Read the model definition and answer for the solid it produces. Units are mm, in the model's axes. A direction names the side the tool comes from. Round coordinates to 2 decimals unless told otherwise and drop trailing zeros. Loops run counter-clockwise (first coordinate to the right, second up) from the corner with the lowest first, then second, coordinate; pieces in that order, holes last. Notation, with made-up numbers: M 69.25,14.5 L 124.25,14.5 A29 cw 124.25,44.5 Z; hole C 58.5,-36 d5. An arc over 180 degrees is marked long. Write each question's results on one line, items separated by ' | '.
from build123d import *

# Parameters (mm, degrees)
SKETCH_1_W                     = 55
SKETCH_1_H                     = 60
EXTRUDE_1_DEPTH                = 16.5
HOLE_WIZARD_3_6_3_6_1_D        = 3.6
HOLE_WIZARD_3_6_3_6_1_DEPTH    = 25
HOLE_WIZARD_3_6_3_6_1_TIP      = 1.081549114
HOLE_WIZARD_M2_5_1_D           = 2.05
HOLE_WIZARD_M2_5_1_DEPTH       = 14
HOLE_WIZARD_M2_5_1_TIP         = 0.615882135
SKETCH_8_W                     = 35
SKETCH_8_H                     = 20.4
CUT_EXTRUDE_1_DEPTH            = 44.914690025
CUT_EXTRUDE_START              = 2.5
SKETCH_9_W                     = 20
SKETCH_9_H                     = 6
CUT_EXTRUDE_2_DEPTH            = 42.414690025
SHELL_START                    = 1.8
SHELL_1_DEPTH                  = 14.7
EXTRUDE_2_DEPTH                = 3
HOLE_WIZARD_1_AT_2_COUNT       = 2
HOLE_WIZARD_1_AT_2_PITCH       = 48
HOLE_WIZARD_1_AT_3_COUNT       = 2
HOLE_WIZARD_1_AT_3_PITCH       = 27.5
HOLE_WIZARD_1_AT_4_COUNT       = 2
HOLE_WIZARD_1_AT_4_PITCH       = 70.507091842
CUT_EXTRUDE_START_2            = -1.5
SKETCH_15_R                    = 5
SKETCH_15_R_2                  = 1.5
CUT_EXTRUDE_3_DEPTH            = 17.5
SKETCH_16_R                    = 3
CUT_EXTRUDE_4_DEPTH            = 12
CUT_EXTRUDE_5_DEPTH            = 45.379499772
CUT_EXTRUDE_5_DEPTH_BACK       = 45.379499772
SKETCH_17_R                    = 5
FILLET_1_R                     = 0.5
FILLET_2_R                     = 0.5
SKETCH_20_W                    = 2
SKETCH_20_H                    = 3
HOLE_WIZARD_4_0_4_1_AT_2_COUNT = 2
HOLE_WIZARD_4_0_4_1_AT_2_PITCH = 27.5
HOLE_WIZARD_4_0_4_1_AT_3_COUNT = 2
HOLE_WIZARD_4_0_4_1_AT_3_PITCH = 61.846584384
HOLE_WIZARD_4_0_4_1_AT_4_COUNT = 2
HOLE_WIZARD_4_0_4_1_AT_4_PITCH = 48
HOLE_WIZARD_2_7_2_7_1_D        = 2.7


# Read off the part's stored shape, not the designer's step: 抽壳1
with BuildPart() as part:
    # 草图1 → 凸台-拉伸1 (new body)
    with BuildSketch(Plane.XY):
        Rectangle(SKETCH_1_W, SKETCH_1_H)
    extrude(amount=EXTRUDE_1_DEPTH)

    # Ø3.6 (3.6) 直径孔1
    with Locations(Plane.XY.offset(16.5)):
        with Locations((-24, 21.5), (24, 21.5), (24, -6), (-15, -26.5)):
            Hole(HOLE_WIZARD_3_6_3_6_1_D / 2, depth=HOLE_WIZARD_3_6_3_6_1_DEPTH)
            with Locations((0, 0, -(HOLE_WIZARD_3_6_3_6_1_DEPTH + HOLE_WIZARD_3_6_3_6_1_TIP / 2))):  # 118° drill point
                Cone(0, HOLE_WIZARD_3_6_3_6_1_D / 2, HOLE_WIZARD_3_6_3_6_1_TIP, mode=Mode.SUBTRACT)

    # M2.5 螺纹孔1
    with Locations(Plane.XY.offset(16.5)):
        with Locations((-24, 26.5), (24, 26.5), (24, -1), (-22.5, -26.5)):
            Hole(HOLE_WIZARD_M2_5_1_D / 2, depth=HOLE_WIZARD_M2_5_1_DEPTH)
            with Locations((0, 0, -(HOLE_WIZARD_M2_5_1_DEPTH + HOLE_WIZARD_M2_5_1_TIP / 2))):  # 118° drill point
                Cone(0, HOLE_WIZARD_M2_5_1_D / 2, HOLE_WIZARD_M2_5_1_TIP, mode=Mode.SUBTRACT)

    # 草图8 → 切除-拉伸1 (cut, through all)
    with BuildSketch(Plane.XY.offset(16.5)):
        with Locations((10, -19.8)):
            Rectangle(SKETCH_8_W, SKETCH_8_H)
    extrude(amount=-CUT_EXTRUDE_1_DEPTH, mode=Mode.SUBTRACT)

    # 草图9 → 切除-拉伸2 (cut, through all)
    with BuildSketch(Plane(origin=(0, 0, 16.5), x_dir=(-1, 0, 0), z_dir=(0, 0, -1)).offset(CUT_EXTRUDE_START)):
        with Locations((17.5, -27)):
            Rectangle(SKETCH_9_W, SKETCH_9_H)
    extrude(amount=CUT_EXTRUDE_2_DEPTH, mode=Mode.SUBTRACT)

    # 抽壳1 outline → 抽壳1 (cut)
    with BuildSketch(Plane.XY.offset(SHELL_START)):
        with BuildLine():
            ThreePointArc((-21.743758657, 28.2), (-21.182110509, 26.299690696), (-22.006919283, 24.4979375))
            ThreePointArc((-22.006919283, 24.4979375), (-20.910890356, 19.651378458), (-25.7, 18.326673669))
            Line((-25.7, 18.326673669), (-25.7, -22.2))
            Line((-25.7, -22.2), (-9.3, -22.2))
            Line((-9.3, -22.2), (-9.3, -7.8))
            Line((-9.3, -7.8), (20.882308546, -7.8))
            ThreePointArc((20.882308546, -7.8), (20.494996561, -5.178446051), (22.006919283, -3.0020625))
            ThreePointArc((22.006919283, -3.0020625), (21.865811165, 0.8509087), (25.7, 1.256241343))
            Line((25.7, 1.256241343), (25.7, 18.326673669))
            ThreePointArc((25.7, 18.326673669), (20.910890356, 19.651378458), (22.006919283, 24.4979375))
            ThreePointArc((22.006919283, 24.4979375), (21.182110509, 26.299690696), (21.743758657, 28.2))
            Line((21.743758657, 28.2), (-21.743758657, 28.2))
        make_face()
    extrude(amount=SHELL_1_DEPTH, mode=Mode.SUBTRACT)


with BuildPart() as body_2:
    # 草图10 → 凸台-拉伸2 (new body)
    with BuildSketch(Plane.XY.offset(16.5)):
        Polygon((-27.5, -30), (-7.5, -30), (-7.5, -9.6), (27.5, -9.6), (27.5, 30), (-27.5, 30), align=None)
    extrude(amount=EXTRUDE_2_DEPTH)


with BuildPart() as hole_wizard_1_tool:
    # 草图13 → 打孔尺寸(%根据)内六角圆柱头螺钉的类型1 (revolve)
    with BuildSketch(Plane(origin=(24, 26.5, 19.5), x_dir=(0, -1, 0), z_dir=(1, 0, 0))):
        Polygon((0, 0), (0, 19.5), (1.1, 19.5), (1.1, 1.8), (2.6, 1.8), (2.6, 0), align=None)
    hole_wizard_1 = revolve(axis=Axis((24, 26.5, 25.85), (0, 0, -1)))


with BuildPart() as part_1:
    add(part.part)

    # 打孔尺寸(%根据)内六角圆柱头螺钉的类型1: cut by hole_wizard_1_tool
    add(hole_wizard_1_tool.part, mode=Mode.SUBTRACT)


with BuildPart() as body_2_1:
    add(body_2.part)

    # 打孔尺寸(%根据)内六角圆柱头螺钉的类型1: cut by hole_wizard_1_tool
    add(hole_wizard_1_tool.part, mode=Mode.SUBTRACT)


with BuildPart() as hole_wizard_1_at_2_tool:
    # 打孔尺寸(%根据)内六角圆柱头螺钉的类型1 at 2: 打孔尺寸(%根据)内六角圆柱头螺钉的类型1 ×2
    with Locations(*[(-i * HOLE_WIZARD_1_AT_2_PITCH, 0, 0) for i in range(1, HOLE_WIZARD_1_AT_2_COUNT)]):
        add(hole_wizard_1)


with BuildPart() as part_2:
    add(part_1.part)

    # 打孔尺寸(%根据)内六角圆柱头螺钉的类型1 at 2: cut by hole_wizard_1_at_2_tool
    add(hole_wizard_1_at_2_tool.part, mode=Mode.SUBTRACT)


with BuildPart() as body_2_2:
    add(body_2_1.part)

    # 打孔尺寸(%根据)内六角圆柱头螺钉的类型1 at 2: cut by hole_wizard_1_at_2_tool
    add(hole_wizard_1_at_2_tool.part, mode=Mode.SUBTRACT)


with BuildPart() as hole_wizard_1_at_3_tool:
    # 打孔尺寸(%根据)内六角圆柱头螺钉的类型1 at 3: 打孔尺寸(%根据)内六角圆柱头螺钉的类型1 ×2
    with Locations(*[(0, -i * HOLE_WIZARD_1_AT_3_PITCH, 0) for i in range(1, HOLE_WIZARD_1_AT_3_COUNT)]):
        add(hole_wizard_1)


with BuildPart() as part_3:
    add(part_2.part)

    # 打孔尺寸(%根据)内六角圆柱头螺钉的类型1 at 3: cut by hole_wizard_1_at_3_tool
    add(hole_wizard_1_at_3_tool.part, mode=Mode.SUBTRACT)


with BuildPart() as body_2_3:
    add(body_2_2.part)

    # 打孔尺寸(%根据)内六角圆柱头螺钉的类型1 at 3: cut by hole_wizard_1_at_3_tool
    add(hole_wizard_1_at_3_tool.part, mode=Mode.SUBTRACT)


with BuildPart() as hole_wizard_1_at_4_tool:
    # 打孔尺寸(%根据)内六角圆柱头螺钉的类型1 at 4: 打孔尺寸(%根据)内六角圆柱头螺钉的类型1 ×2
    with Locations(*[Vector(-0.6595081258531857, -0.7516974337681476, 0) * (i * HOLE_WIZARD_1_AT_4_PITCH) for i in range(1, HOLE_WIZARD_1_AT_4_COUNT)]):
        add(hole_wizard_1)


with BuildPart() as part_4:
    add(part_3.part)

    # 打孔尺寸(%根据)内六角圆柱头螺钉的类型1 at 4: cut by hole_wizard_1_at_4_tool
    add(hole_wizard_1_at_4_tool.part, mode=Mode.SUBTRACT)


with BuildPart() as body_2_4:
    add(body_2_3.part)

    # 打孔尺寸(%根据)内六角圆柱头螺钉的类型1 at 4: cut by hole_wizard_1_at_4_tool
    add(hole_wizard_1_at_4_tool.part, mode=Mode.SUBTRACT)


with BuildPart() as cut_extrude_3_tool:
    # 草图15 → 切除-拉伸3 (new body)
    with BuildSketch(Plane.XY.offset(1.8).offset(CUT_EXTRUDE_START_2)):
        with Locations((6.5, 9.5)):
            Circle(SKETCH_15_R)
        with Locations((-12.549056621, 13.669345493)):
            Circle(SKETCH_15_R_2)
        with Locations((-17, 1.988630488)):
            Circle(SKETCH_15_R_2)
        with Locations((-17.5, -9)):
            Circle(SKETCH_15_R_2)
    extrude(amount=CUT_EXTRUDE_3_DEPTH)


with BuildPart() as part_5:
    add(part_4.part)

    # 切除-拉伸3: cut by cut_extrude_3_tool
    add(cut_extrude_3_tool.part, mode=Mode.SUBTRACT)

    # 草图16 → 切除-拉伸4 (cut)
    with BuildSketch(Plane(origin=(-7.5, 0, 0), x_dir=(0, 0, -1), z_dir=(1, 0, 0))):
        with Locations(Location((-8, -18, 0), (0, 0, 90))):
            Circle(SKETCH_16_R)
    extrude(amount=-CUT_EXTRUDE_4_DEPTH, mode=Mode.SUBTRACT)


with BuildPart() as body_2_5:
    add(body_2_4.part)

    # 切除-拉伸3: cut by cut_extrude_3_tool
    add(cut_extrude_3_tool.part, mode=Mode.SUBTRACT)


with BuildPart() as cut_extrude_5_tool:
    # 草图17 → 切除-拉伸5 (new, two sides: drawn at the far end of the back side and taken through both)
    with BuildSketch(Plane.XY.offset(1.8).offset(-CUT_EXTRUDE_5_DEPTH_BACK)):
        with Locations((6.5, 9.5)):
            Circle(SKETCH_17_R)
    extrude(amount=CUT_EXTRUDE_5_DEPTH + CUT_EXTRUDE_5_DEPTH_BACK)


with BuildPart() as part_6:
    add(part_5.part)

    # 切除-拉伸5: cut by cut_extrude_5_tool
    add(cut_extrude_5_tool.part, mode=Mode.SUBTRACT)

    # 圆角1
    fillet_1_edges = [part_6.edges().sort_by_distance(p)[0] for p in [
        (-27.5, 3, 0),
        (0, 30, 0),
        (27.5, 10.2, 0),
        (27.5, -9.6, 8.25),
        (-7.5, -16.8, 0),
        (10, -9.6, 0),
        (-7.5, -9.6, 8.25),
        (-7.5, -30, 15.25),
        (-27.5, -30, 15.25),
        (-27.5, 30, 8.25),
        (27.5, 30, 8.25),
        (-17.5, -24, 0),
        (-7.5, -24, 7),
        (-27.5, -24, 7),
    ]]
    fillet(fillet_1_edges, radius=FILLET_1_R)


with BuildPart() as body_2_6:
    add(body_2_5.part)

    # 切除-拉伸5: cut by cut_extrude_5_tool
    add(cut_extrude_5_tool.part, mode=Mode.SUBTRACT)

    # 圆角2
    fillet_2_edges = [body_2_6.edges().sort_by_distance(p)[0] for p in [
        (-27.5, 30, 18),
        (27.5, 30, 18),
        (27.5, -9.6, 18),
        (-7.5, -9.6, 18),
        (-7.5, -30, 18),
        (-27.5, -30, 18),
    ]]
    fillet(fillet_2_edges, radius=FILLET_2_R)

    # 草图20 → Ø4.0 (4) 直径孔1 (revolve, cut)
    with BuildSketch(Plane(origin=(24, 21.5, 16.5), x_dir=(0, 1, 0), z_dir=(1, 0, 0))):
        with Locations((1, 1.5)):
            Rectangle(SKETCH_20_W, SKETCH_20_H)
    hole_wizard_4_0_4_1 = revolve(axis=Axis((24, 21.5, 10.15), (0, 0, 1)), mode=Mode.SUBTRACT)

    # Ø4.0 (4) 直径孔1 at 2: Ø4.0 (4) 直径孔1 ×2
    with Locations(*[(0, -i * HOLE_WIZARD_4_0_4_1_AT_2_PITCH, 0) for i in range(1, HOLE_WIZARD_4_0_4_1_AT_2_COUNT)]):
        add(hole_wizard_4_0_4_1, mode=Mode.SUBTRACT)

    # Ø4.0 (4) 直径孔1 at 3: Ø4.0 (4) 直径孔1 ×2
    with Locations(*[Vector(-0.6305926250944656, -0.7761140001162656, 0) * (i * HOLE_WIZARD_4_0_4_1_AT_3_PITCH) for i in range(1, HOLE_WIZARD_4_0_4_1_AT_3_COUNT)]):
        add(hole_wizard_4_0_4_1, mode=Mode.SUBTRACT)

    # Ø4.0 (4) 直径孔1 at 4: Ø4.0 (4) 直径孔1 ×2
    with Locations(*[(-i * HOLE_WIZARD_4_0_4_1_AT_4_PITCH, 0, 0) for i in range(1, HOLE_WIZARD_4_0_4_1_AT_4_COUNT)]):
        add(hole_wizard_4_0_4_1, mode=Mode.SUBTRACT)

    # Ø2.7 (2.7) 直径孔1 (through all)
    with Locations(Plane.XY.offset(17.7)):
        with Locations((24, 26.5), (24, -1), (-24, 26.5), (-22.5, -26.5)):
            Hole(HOLE_WIZARD_2_7_2_7_1_D / 2)


solid = body_2_6.part
Item 1: The part is cut by section A-A (y = -26.5). Determine the outline of the cut face in (x, z), plus the area to 3 significant figures.
Outcome:
outline: M -27.5,16.5 L -23.85,16.5 L -23.85,17.7 L -25.1,17.7 L -25.1,19.5 L -27.5,19.5 Z; M -21.15,16.5 L -17,16.5 L -17,19.5 L -19.9,19.5 L -19.9,17.7 L -21.15,17.7 Z; M -13,16.5 L -7.5,16.5 L -7.5,19.5 L -13,19.5 Z | area: 35.4 mm2
Item 2: The mould has two halves that part along X. Classify faces 4 (the face through (-18, -9, 17.8)), 5 (the face through (10, -9.6, 18)): pulls with the +X half, pulls with the -X half, needs draft (parallel to the pull), parting line crosses it, or undercut.
Outcome:
face 4: undercut | face 5: needs draft
Item 3: The part is cut by section B-B (x = 24). Determine the outline of the cut face in (y, z), plus the area to 3 significant figures.
Outcome:
outline: M -9.6,16.5 L -8,16.5 L -8,19.5 L -9.6,19.5 Z; M -4,16.5 L -2.35,16.5 L -2.35,17.7 L -3.6,17.7 L -3.6,19.5 L -4,19.5 Z; M 0.35,16.5 L 19.5,16.5 L 19.5,19.5 L 1.6,19.5 L 1.6,17.7 L 0.35,17.7 Z; M 23.5,16.5 L 25.15,16.5 L 25.15,17.7 L 23.9,17.7 L 23.9,19.5 L 23.5,19.5 Z; M 27.85,16.5 L 30,16.5 L 30,19.5 L 29.1,19.5 L 29.1,17.7 L 27.85,17.7 Z | area: 69.6 mm2
Item 4: Flat-ended cylindrical pins translate along their axes: pin 1 (1.5 mm diameter, centred on x = 10.5, z = 18, fed in from -Y); pin 2 (1.5 mm diameter, centred on x = -18, y = -9.5, fed in from -Z); pin 3 (2.5 mm diameter, centred on x = 23.5, y = -2, fed in from +Z); pin 4 (9 mm diameter, centred on x = 6.5, y = 9.5, fed in from -Z). Find the tip coordinate at first contact, or state that the pin passes through.
Outcome:
pin 1: stops at y = -9.6 | pin 2: stops at z = 17.8 | pin 3: stops at z = 17.7 | pin 4: passes through
Item 5: For faces 1 (the face through (23.38, 25.3, 17.09)), 2 (the face through (-19, -9, 17)), 3 (the face through (21.422, -0.662, 18.613)), determine the directions among +Z, -Z, +X, -X, +Y, -Y from which every point of the face is accessible in a straight line to the end or side of a thin tool.
Outcome:
face 1: +Z, -Z | face 2: -Z | face 3: +Z
Item 6: The part is cut by section D-D (y = -6). Determine the outline of the cut face in (x, z).
Outcome:
outline: M -27.5,16.5 L 22,16.5 L 22,19.5 L -27.5,19.5 Z; M 26,16.5 L 27.5,16.5 L 27.5,19.5 L 26,19.5 Z
Item 7: Straight lines are drawn through the part: line 1 (Y direction, x = 24, z = 16.9); line 2 (Y direction, x = 24, z = 18.7); line 3 (X direction, y = -26.5, z = 18.35). For each, find the intervals that lie inside material, in ascending order.
Outcome:
line 1: y = -9.6 to -8, -4 to -2.35, 0.35 to 19.5, 23.5 to 25.15, 27.85 to 30 | line 2: y = -9.6 to -8, -4 to -3.6, 1.6 to 19.5, 23.5 to 23.9, 29.1 to 30 | line 3: x = -27.5 to -25.1, -19.9 to -17, -13 to -7.5
Item 8: The part is cut by section C-C (z = 18.4). State how many separate pieces and enclosed holes the cut face has, plus the area to 3 significant figures.
Outcome:
separate pieces: 1 | enclosed holes: 9 | area: 2,370 mm2
